The model under review builds one solid part; all positions refer to its coordinate system, in mm. A direction names the side the tool comes from. Coordinates: 2 decimals unless noted, no trailing zeros. Write each loop counter-clockwise with the first axis right and the second up, starting at its lowest first coordinate (ties: lowest second). Pieces come first, ordered by that corner, then holes. Notation, with made-up numbers: (15.25, -18) - (30.25, -18) arc R19 cw to (30.25, 19) - close; hole circle Ø8 at (31.25, 71). An arc over 180 degrees is marked (long way). Put each result on its own line as item: value.
from build123d import *

# Parameters (mm, degrees)
BOSS_EXTRUDE1_DEPTH     = 580
CUT_EXTRUDE1_DEPTH      = 3
TAP_DRILL_FOR_M3_TAP1_D = 2.5
M5_CLEARANCE_HOLE1_D    = 5.5


with BuildPart() as part:
    # Sketch1 → Boss-Extrude1 (new body)
    with BuildSketch(Plane.XY):
        Polygon((0, 0), (0, 40), (40, 40), (40, 36), (4, 36), (4, 0), align=None)
    extrude(amount=BOSS_EXTRUDE1_DEPTH)

    # Sketch2 → Cut-Extrude1 (cut)
    with BuildSketch(Plane(origin=(0, 36, 0), x_dir=(1, 0, 0), z_dir=(0, 1, 0))):
        Polygon((24.309401077, -14.924264069), (19.690598923, -14.924264069), (17.381197846, -18.924264069), (19.690598923, -22.924264069), (24.309401077, -22.924264069), (26.618802154, -18.924264069), align=None)
        Polygon((24.309401077, -557.075735931), (19.690598923, -557.075735931), (17.381197846, -561.075735931), (19.690598923, -565.075735931), (24.309401077, -565.075735931), (26.618802154, -561.075735931), align=None)
    extrude(amount=CUT_EXTRUDE1_DEPTH, mode=Mode.SUBTRACT)

    # Tap Drill for M3 Tap1 (through all)
    with Locations(Plane(origin=(0, 40, 0), x_dir=(1, 0, 0), z_dir=(0, 1, 0))):
        with Locations((22, -549.075735931), (22, -573.075735931), (22, -30.924264069), (22, -6.924264069)):
            Hole(TAP_DRILL_FOR_M3_TAP1_D / 2)

    # M5 Clearance Hole1 (through all)
    with Locations(Plane(origin=(0, 39, 0), x_dir=(-1, 0, 0), z_dir=(0, -1, 0))):
        with Locations((-22, -561.075735931), (-22, -18.924264069)):
            Hole(M5_CLEARANCE_HOLE1_D / 2)


solid = part.part
1. Consider section C-C on y = 13. State the section outline as (x, z) points.
Determined:
outline: (0, 0) - (4, 0) - (4, 580) - (0, 580) - close
2. Machinability: for faces 1 (the flat face through (0, 20, 286)), 2 (the flat face through (22, 36, 286)), which of the approach directions +Z, -Z, +X, -X, +Y, -Y give a long, thin tool a straight path to every point of the face, cutting with its end or side? Answer none if there is none.
Determined:
face 1: +Z, -Z, -X, +Y, -Y
face 2: +Z, -Z, +X, -Y
3. For pin 1 Ø9 at (x, z) = (22, 18.92) entering from +Y; pin 2 Ø4.5 at (x, z) = (22, 561.08) entering from -Y; pin 3 Ø18 at (x, z) = (29, 259) entering from -Y; pin 4 Ø12 at (y, z) = (5, 514.5) entering from +X, all flat-tipped, find the tip position at first contact; note any pin that passes through.
Determined:
pin 1: stops at y = 40
pin 2: passes through
pin 3: stops at y = 36
pin 4: stops at x = 4
4. To check wall thickness, follow probe 1 along Y at (x, z) = (26, 142); probe 2 along X at (y, z) = (14, 392.5); probe 3 along X at (y, z) = (37.5, 30.5). State the ranges of each line that lie inside material, in increasing order.
Determined:
probe 1: y = 36 to 40
probe 2: x = 0 to 4
probe 3: x = 0 to 20.82, 23.18 to 40
5. Consider section B-B on x = 32.5. State the section outline as (y, z) points, plus the area to 3 significant figures.
Determined:
outline: (36, 0) - (40, 0) - (40, 580) - (36, 580) - close
area: 2,320 mm^2
6. Consider section A-A on z = 273. State the section outline as (x, y) points, plus the area to 3 significant figures.
Determined:
outline: (0, 0) - (4, 0) - (4, 36) - (40, 36) - (40, 40) - (0, 40) - close
area: 304 mm^2
